```python
from build123d import *

# Parameters (mm, degrees)
SKETCH1_W           = 38.1
SKETCH1_H           = 88.9
BOSS_EXTRUDE1_DEPTH = 2362.2
SKETCH2_R           = 21.43125
CUT_EXTRUDE4_DEPTH  = 918.6545
SKETCH3_R           = 4.7625
CUT_EXTRUDE5_DEPTH  = 2363.925359062
FILLET1_R           = 3.175


with BuildPart() as part:
    # Sketch1 → Boss-Extrude1 (new body)
    with BuildSketch(Plane(origin=(0, 0, 0), x_dir=(1, 0, 0), z_dir=(0, 1, 0))):
        Rectangle(SKETCH1_W, SKETCH1_H)
    extrude(amount=BOSS_EXTRUDE1_DEPTH)

    # Sketch2 → Cut-Extrude4 (cut)
    with BuildSketch(Plane(origin=(19.05, 0, 0), x_dir=(0, 0, -1), z_dir=(1, 0, 0))):
        with Locations((12.7, 458.7875)):
            Circle(SKETCH2_R)
        with Locations((12.7, 939.8)):
            Circle(SKETCH2_R)
        with Locations((12.7, 1420.84425)):
            Circle(SKETCH2_R)
        with Locations((12.7, 1901.8885)):
            Circle(SKETCH2_R)
    extrude(amount=-CUT_EXTRUDE4_DEPTH, mode=Mode.SUBTRACT)

    # Sketch3 → Cut-Extrude5 (cut, through all)
    with BuildSketch(Plane(origin=(19.05, 0, 0), x_dir=(0, 0, -1), z_dir=(1, 0, 0))):
        with Locations((-33.3375, 112.7125)):
            Circle(SKETCH3_R)
        with Locations((-33.3375, 608.0125)):
            Circle(SKETCH3_R)
        with Locations((-33.3375, 1103.3125)):
            Circle(SKETCH3_R)
    cut_extrude5 = extrude(amount=-CUT_EXTRUDE5_DEPTH, mode=Mode.SUBTRACT)

    # Fillet1
    fillet1_edges = [part.edges().sort_by_distance(p)[0] for p in [
        (19.05, 1181.1, 44.45),
        (-19.05, 1181.1, 44.45),
        (-19.05, 1181.1, -44.45),
        (19.05, 1181.1, -44.45),
    ]]
    fillet(fillet1_edges, radius=FILLET1_R)

    # Mirror1: Cut-Extrude5 across plane
    add(cut_extrude5.mirror(Plane.ZX.offset(1181.1)), mode=Mode.SUBTRACT)


solid = part.part
```
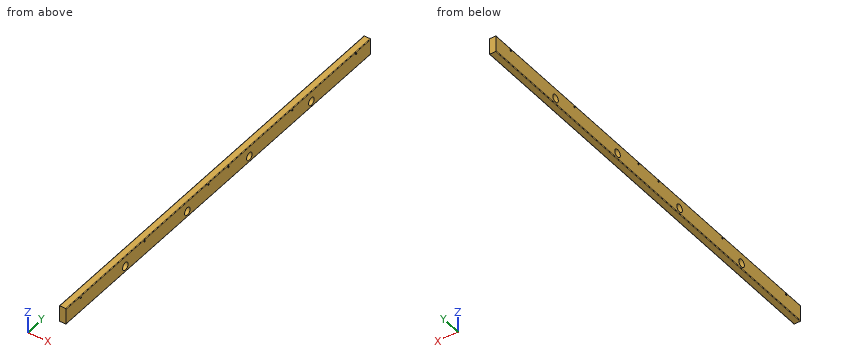
For this review, take the finished solid that the model builds, in its own axes (mm). Round coordinates to 2 decimals unless told otherwise and drop trailing zeros. Loops run counter-clockwise (first coordinate to the right, second up) from the corner with the lowest first, then second, coordinate; pieces in that order, holes last.
Q1. To check wall thickness, follow line 1 along Y through (x, z) = (0, -12.7); line 2 along Y through (x, z) = (12, -10.5); line 3 along Z through (x, y) = (-9, 939). State the ranges of each line that lie inside material, in increasing order.
Result sheet:
line 1: y = 0 to 437.36, 480.22 to 918.37, 961.23 to 1399.41, 1442.28 to 1880.46, 1923.32 to 2362.2
line 2: y = 0 to 437.47, 480.11 to 918.48, 961.12 to 1399.53, 1442.16 to 1880.57, 1923.21 to 2362.2
line 3: z = -44.45 to -34.12, 8.72 to 44.45
Q2. Add section A-A on z = -12.7. Write out the cut boundary in (x, y).
Result sheet:
outline: (-19.05, 0) - (19.05, 0) - (19.05, 437.36) - (-19.05, 437.36) - close; (-19.05, 480.22) - (19.05, 480.22) - (19.05, 918.37) - (-19.05, 918.37) - close; (-19.05, 961.23) - (19.05, 961.23) - (19.05, 1399.41) - (-19.05, 1399.41) - close; (-19.05, 1442.28) - (19.05, 1442.28) - (19.05, 1880.46) - (-19.05, 1880.46) - close; (-19.05, 1923.32) - (19.05, 1923.32) - (19.05, 2362.2) - (-19.05, 2362.2) - close
Q3. Add section C-C on x = -3. Give the number of separate pieces and of enclosed holes in the cut face, plus the area to 3 significant figures.
Result sheet:
separate pieces: 1
enclosed holes: 10
area: 204,000 mm2
Q4. Add section B-B on y = 939.8. Write out the cut boundary in (x, z) (3 decimals), plus the area to 3 significant figures.
Result sheet:
outline: (-19.05, -41.275) arc R3.175 ccw to (-15.875, -44.45) - (15.875, -44.45) arc R3.175 ccw to (19.05, -41.275) - (19.05, -34.131) - (-19.05, -34.131) - close; (-19.05, 8.731) - (19.05, 8.731) - (19.05, 41.275) arc R3.175 ccw to (15.875, 44.45) - (-15.875, 44.45) arc R3.175 ccw to (-19.05, 41.275) - close
area: 1,750 mm2
Q5. Insertion check: pin 1 Ø5.5 at (y, z) = (2249.49, 33.34) entering from +X. The pin has a flat end and moves straight along its axis. Give the tip position at first contact, or say it passes through.
Result sheet:
pin 1: passes through
